Input: part model. Units: mm. Frame: model coordinates. A direction names the side the tool comes from. Round coordinates to 2 decimals unless told otherwise and drop trailing zeros. Loops run counter-clockwise (first coordinate to the right, second up) from the corner with the lowest first, then second, coordinate; pieces in that order, holes last. Notation, with made-up numbers: M -3.75,66.25 L 5.25,66.25 A23 ccw 5.25,89.25 Z; hole C 54,-27.75 d9. An arc over 180 degrees is marked long. Use one line per item in the form item = value. Start each with the question number.
Q1. Mould query, pull axis X, two halves, no side actions, for faces 1 (the flat face through (0, -13, 6.032)), 2 (the flat face through (0, -18, -8.572)), 3 (the flat face through (-8.572, -18, 0)), 4 (the cylindrical face through (7.618, 17.456, -7.667)). Classes: pulls with the +X half, pulls with the -X half, needs draft (parallel to the pull), parting line crosses it, or undercut.
Q2. First-contact query: P1, Ø4, axis at x = -1, y = -20.5, coming from the -Z side; P2, Ø6, axis at x = -1, y = -26.5, coming from the +Z side; P3, Ø1.3, axis at y = -7, z = 7, coming from the -X side; P4, Ø1.8, axis at x = 0, y = 0, coming from the +Z side. Flat tips, straight axial feed; report the tip coordinate or a pass-through.
Q3. Ray query, line 1 along Z through (x, y) = (0, 2); line 2 along Y through (x, z) = (0, -5.75); line 3 along X through (y, z) = (0, 7.25). Return the intervals inside material, ascending.
Q4. Access query for faces 5 (the cylindrical face through (7.618, -17.85, -7.667)), 6 (the flat face through (0, 17, 8.572)), 7 (the flat face through (0.06, -28.38, 7.32)), 8 (the flat face through (0, 17, -8.572)). Directions: +Z, -Z, +X, -X, +Y, -Y. A direction counts if a zero-diameter tool reaches every point of the face in a straight line with its end or side. Return the directions, or none.
Q5. Section query C-C, the plane y = 0. Output: boundary loops of the cut face in (x, z) (1 decimal).
Q6. Section query A-A, the plane z = 0. Output: boundary loops of the cut face in (x, y), and give its area (3 significant figures).
Q7. Section query D-D, the plane z = 3.25. Output: boundary loops of the cut face in (x, y).
Autodesk Inventor part; units mm, degrees
ref_plane "YZ Plane" through (0, 0, 0) normal (1, 0, 0) x (0, 1, 0)
ref_plane "XZ Plane" through (0, 0, 0) normal (0, 1, 0) x (-1, 0, 0)
ref_plane "XY Plane" through (0, 0, 0) normal (0, 0, 1) x (1, 0, 0)
sketch "Sketch1" plane through (0, 0, 0) normal (0, 1, 0) x (-1, 0, 0)
  line L0 (11.43, 11.43) -> (-11.43, 11.43)
  line L1 (-11.43, 11.43) -> (-11.43, -11.43)
  line L2 (-11.43, -11.43) -> (11.43, -11.43)
  line L3 (11.43, -11.43) -> (11.43, 11.43)
  line L4 (11.43, 11.43) -> (-11.43, -11.43) construction
  line L5 (-11.43, 11.43) -> (11.43, -11.43) construction
  point P0 (0, 0)
  dimension "outerWidth" = 22.86
  dimension "outerLength" = 22.86
extrude "Extrusion1" add sketch "Sketch1" along normal mid plane 7.112
sketch "Sketch2" plane through (0, 0, 0) normal (0, 1, 0) x (-1, 0, 0)
  line L0 (8.5725, 8.5725) -> (-8.5725, 8.5725)
  line L1 (-8.5725, 8.5725) -> (-8.5725, -8.5725)
  line L2 (-8.5725, -8.5725) -> (8.5725, -8.5725)
  line L3 (8.5725, -8.5725) -> (8.5725, 8.5725)
  line L4 (8.5725, 8.5725) -> (-8.5725, -8.5725) construction
  line L5 (-8.5725, 8.5725) -> (8.5725, -8.5725) construction
  point P0 (0, 0)
  dimension "innerWidth" = 17.145
  dimension "innerLength" = 17.145
extrude "Extrusion2" add sketch "Sketch2" along normal mid plane 63.5
sketch "Sketch3" plane through (-8.5725, -3.556, 8.5725) normal (0, 0, 1) x (1, 0, 0)
  line L0 (0, -28.194) -> (17.145, -28.194) construction
  line L1 (13.0175, -28.194) -> (13.0175, 0) construction
  line L2 (20.0025, 0) -> (-2.8575, 0) construction
  line L3 (17.145, 0) -> (17.145, -28.194)
  line L4 (4.1275, -18.9779) -> (13.0175, -22.0396)
  line L5 (13.0175, -22.0396) -> (13.0175, -23.3148)
  line L6 (13.0175, -23.3148) -> (4.1275, -26.3766)
  line L7 (4.1275, -26.3766) -> (4.1275, -25.1086)
  line L8 (4.1275, -25.1086) -> (11.5118, -22.6448)
  line L9 (11.5118, -22.6448) -> (4.1275, -20.181)
  line L10 (4.1275, -20.181) -> (4.1275, -18.9779)
  spline S0 degree 2 poles (8.5725, -8.928) (10.9643, -8.928) (13.2048, -10.3184) (13.2048, -11.7664) knots 0 0 0 1 2 2 2
  spline S1 degree 2 poles (13.2048, -11.7664) (13.2048, -13.2361) (10.9211, -14.6121) (8.5797, -14.6121) knots 0 0 0 1 2 2 2
  spline S2 degree 2 poles (8.5797, -14.6121) (6.1735, -14.6121) (3.9474, -13.2217) (3.9474, -11.7664) knots 0 0 0 1 2 2 2
  spline S3 degree 2 poles (3.9474, -11.7664) (3.9474, -10.304) (6.2527, -8.928) (8.5725, -8.928) knots 0 0 0 1 2 2 2
  spline S4 degree 2 poles (11.2813, -10.4553) (10.8418, -10.2824) (9.4874, -10.1383) (8.5725, -10.1383) knots 0 0 0 1 2 2 2
  spline S5 degree 2 poles (8.5725, -10.1383) (7.6576, -10.1383) (6.3104, -10.2824) (5.8565, -10.4625) knots 0 0 0 1 2 2 2
  spline S6 degree 2 poles (5.8565, -10.4625) (5.4026, -10.6426) (4.9344, -11.2693) (4.9344, -11.7664) knots 0 0 0 1 2 2 2
  spline S7 degree 2 poles (4.9344, -11.7664) (4.9344, -12.2635) (5.4026, -12.9047) (5.8709, -13.092) knots 0 0 0 1 2 2 2
  spline S8 degree 2 poles (5.8709, -13.092) (6.3248, -13.2721) (7.708, -13.4018) (8.5797, -13.4018) knots 0 0 0 1 2 2 2
  spline S9 degree 2 poles (8.5797, -13.4018) (9.5163, -13.4018) (10.7698, -13.2865) (11.2597, -13.0992) knots 0 0 0 1 2 2 2
  spline S10 degree 2 poles (11.2597, -13.0992) (11.7207, -12.9263) (12.2178, -12.2851) (12.2178, -11.7664) knots 0 0 0 1 2 2 2
  spline S11 degree 2 poles (12.2178, -11.7664) (12.2178, -11.2766) (11.7496, -10.6354) (11.2813, -10.4553) knots 0 0 0 1 2 2 2
  line L11 (9.9629, -2.0696) -> (9.9629, -3.1286)
  line L12 (9.9629, -3.1286) -> (13.0175, -3.1286)
  line L13 (13.0175, -3.1286) -> (13.0175, -4.2741)
  line L14 (13.0175, -4.2741) -> (9.9629, -4.2741)
  line L15 (9.9629, -4.2741) -> (9.9629, -8.2004)
  line L16 (9.9629, -8.2004) -> (8.7094, -8.2004)
  line L17 (8.7094, -8.2004) -> (4.1275, -4.2236)
  line L18 (4.1275, -4.2236) -> (4.1275, -3.1286)
  line L19 (4.1275, -3.1286) -> (9.0048, -3.1286)
  line L20 (9.0048, -3.1286) -> (9.0048, -2.0696)
  line L21 (9.0048, -2.0696) -> (9.9629, -2.0696)
  line L22 (9.0048, -4.2741) -> (5.5323, -4.2741)
  line L23 (5.5323, -4.2741) -> (9.0048, -7.2638)
  line L24 (9.0048, -7.2638) -> (9.0048, -4.2741)
  point P0 (8.5725, 3.556)
  dimension "textCenterLine" = 4.1275
extrude "Extrusion4" cut sketch "Sketch3" against normal blind 2.54
sketch "Sketch4" plane through (0, 31.75, 0) normal (0, 1, 0) x (1, 0, 0)
  point P0 (0, 0)
  point P1 (0, 0)
hole "Hole1" at (0, 31.75, 0) direction (0, -1, 0) diameter 9.525 end through all
fillet "Fillet1" radius 1.5875 4 edges at (-11.43, 0, 11.43) (11.43, 0, 11.43) (11.43, 0, -11.43) (-11.43, 0, -11.43)
fillet "Fillet2" radius 3.175 8 edges at (8.5725, 17.653, -8.5725) (8.5725, 17.653, 8.5725) (-8.5725, 17.653, -8.5725) (-8.5725, 17.653, 8.5725) (8.5725, -17.653, -8.5725) (8.5725, -17.653, 8.5725) (-8.5725, -17.653, -8.5725) (-8.5725, -17.653, 8.5725)
sketch "Sketch5" plane through (-9.8425, 3.556, 11.43) normal (0, 0, 1) x (1, 0, 0)
  point P0 (9.8425, -3.556)
  point P1 (9.8425, -3.556)
sketch "Sketch6" plane through (11.43, -3.556, -9.8425) normal (1, 0, 0) x (0, 0, -1)
  point P0 (-9.8425, 3.556)
  point P1 (-9.8425, 3.556)
sketch "Sketch7" plane through (9.8425, 3.556, -11.43) normal (0, 0, -1) x (-1, 0, 0)
  point P0 (9.8425, -3.556)
  point P1 (9.8425, -3.556)
sketch "Sketch8" plane through (-11.43, -3.556, -9.8425) normal (-1, 0, 0) x (0, 0, 1)
  point P0 (9.8425, 3.556)
  point P1 (9.8425, 3.556)
hole "Hole2" at (0, 0, 11.43) direction (0, 0, -1) diameter 3.048 depth 12.7 tip angle 118
hole "Hole3" at (11.43, 0, 0) direction (-1, 0, 0) diameter 3.048 depth 12.7 tip angle 118
hole "Hole4" at (0, 0, -11.43) direction (0, 0, 1) diameter 3.048 depth 12.7 tip angle 118
hole "Hole5" at (-11.43, 0, 0) direction (1, 0, 0) diameter 3.048 depth 12.7 tip angle 118
equation "\"textCenterLine\" = 0.5 * innerWidth - 0.5 * textHeight"
equation "\"textHeight\" = 8.89"
properties part number "Supports"
Results found:
q1.face_1 = undercut
q1.face_2 = needs draft
q1.face_3 = pulls with the -X half
q1.face_4 = pulls with the +X half
q2.P1 = -8.57
q2.P2 = 8.57
q2.P3 = -8.43
q2.P4 = through
q3.line_1 = -11.43 to -4.76, 4.76 to 11.43
q3.line_2 = -31.75 to -1.52, 1.52 to 31.75
q3.line_3 = -11.43 to -1.52, 1.52 to 11.43
q4.face_5 = -Z, +X, -Y
q4.face_6 = +Z, +X, -X, +Y
q4.face_7 = +Z
q4.face_8 = -Z, +X, -X, +Y
q5.outline = M -11.4,-9.8 A1.6 ccw -9.8,-11.4 L -1.5,-11.4 L -1.5,-4.5 A4.8 cw -4.5,-1.5 L -11.4,-1.5 Z; M -11.4,1.5 L -4.5,1.5 A4.8 cw -1.5,4.5 L -1.5,11.4 L -9.8,11.4 A1.6 ccw -11.4,9.8 Z; M 1.5,-11.4 L 9.8,-11.4 A1.6 ccw 11.4,-9.8 L 11.4,-1.5 L 4.5,-1.5 A4.8 cw 1.5,-4.5 Z; M 1.5,4.5 A4.8 cw 4.5,1.5 L 11.4,1.5 L 11.4,9.8 A1.6 ccw 9.8,11.4 L 1.5,11.4 Z
q6.outline = M -11.43,-3.56 L -8.57,-3.56 L -8.57,-31.75 L -4.76,-31.75 L -4.76,-1.52 L -11.43,-1.52 Z; M -11.43,1.52 L -4.76,1.52 L -4.76,31.75 L -8.57,31.75 L -8.57,3.56 L -11.43,3.56 Z; M 4.76,-31.75 L 8.57,-31.75 L 8.57,-3.56 L 11.43,-3.56 L 11.43,-1.52 L 4.76,-1.52 Z; M 4.76,1.52 L 11.43,1.52 L 11.43,3.56 L 8.57,3.56 L 8.57,31.75 L 4.76,31.75 Z
q6.area = 484 mm²
q7.outline = M -11.43,-3.56 L -8.57,-3.56 L -8.57,-31.75 L -3.48,-31.75 L -3.48,31.75 L -8.57,31.75 L -8.57,3.56 L -11.43,3.56 Z; M 3.48,-31.75 L 8.57,-31.75 L 8.57,-3.56 L 11.43,-3.56 L 11.43,3.56 L 8.57,3.56 L 8.57,31.75 L 3.48,31.75 Z
